Read the model definition and answer for the solid it produces. Units are mm, in the model's axes. A direction names the side the tool comes from. Coordinates: 2 decimals unless noted, no trailing zeros. Write each loop counter-clockwise with the first axis right and the second up, starting at its lowest first coordinate (ties: lowest second). Pieces come first, ordered by that corner, then holes. Notation, with made-up numbers: (12.5, 83.5) -> (42.5, 83.5) arc R5 cw to (42.5, 90.5) -> close; hole circle Ø3 at (-12.75, 77). An arc over 180 degrees is marked (long way). Answer as a JSON object with one key per item and string values. Group by question number.
(1) For a pull along Y with two mould halves and no side action, classify faces 4 (the face through (150.266, 29.026, 67.55)), 5 (the face through (150, 660.4, 89)), 6 (the face through (304.8, 326, 84)) as +Y half, -Y half, draft (parallel to the pull), parting line (faces both ways), or undercut.
(2) Which of the six approach directions +Z, -Z, +X, -X, +Y, -Y give full straight-line access (tool end or side, diameter ignored) to faces 1 (the face through (150.266, 273.576, 66.708)), 2 (the face through (150, 13, 56.872)), 3 (the face through (150, 585, 69.85))?
(3) Straight lines are drawn through the part: L1, parallel to Y at x = 57.5, z = 60; L2, parallel to Z at x = 71, y = 619; L3, parallel to Y at x = 237, z = 50. For each, find the intervals that lie inside material, in ascending order.
(4) Flat-ended cylindrical pins translate along their axes: P1, Ø1.5, axis at x = 97, z = 37.5, coming from the -Y side; P2, Ø1.5, axis at x = 111.5, z = 45.5, coming from the -Y side; P3, Ø20.5, axis at x = 89.5, y = 18, coming from the -Z side. Find the tip coordinate at first contact, or state that the pin passes through.
(5) Find section B-B (y = 566). Give the vertices of the cut face in (x, z).
(6) Find section A-A (x = 264.5). Give the vertices of the cut face in (y, z), then the cut area to 3 significant figures.
(7) Find section C-C (z = 44.5). Give the vertices of the cut face in (x, y), then the cut area to 3 significant figures.
from build123d import *

# Parameters (mm, degrees)
F1_W     = 660.4
F1_H     = 107.95
F2_DEPTH = 304.8
F3_DEPTH = 304.801


with BuildPart() as f2:
    # F1 (on Right) → F2 (new body)
    with BuildSketch(Plane.YZ):
        with Locations((330.2, 53.975)):
            Rectangle(F1_W, F1_H)
    extrude(amount=F2_DEPTH)

    # F0 (on Right) → F3 (cut, through all)
    with BuildSketch(Plane.YZ):
        with BuildLine():
            Line((0, 0), (25.4, 0))
            Line((25.4, 0), (635, 0))
            Line((635, 0), (660.4, 0))
            Line((660.4, 0), (660.4, 69.85))
            Line((660.4, 69.85), (635, 69.85))
            Line((635, 69.85), (508, 69.85))
            ThreePointArc((508, 69.85), (501.120084, 68.473081), (495.3, 64.554436))
            ThreePointArc((495.3, 64.554436), (387.828804, 19.05896), (279.4, 62.222496))
            ThreePointArc((279.4, 62.222496), (273.485985, 66.762175), (266.7, 69.85))
            ThreePointArc((266.7, 69.85), (152.689214, 88.843713), (38.1, 73.726423))
            ThreePointArc((38.1, 73.726423), (28.93043, 67.423949), (25.4, 56.872255))
            Line((25.4, 56.872255), (0, 56.872255))
            Line((0, 56.872255), (0, 0))
        make_face()
    extrude(amount=F3_DEPTH, mode=Mode.SUBTRACT)


solid = f2.part
Results below:
{
 "1": {"face 4": "undercut", "face 5": "+Y half", "face 6": "draft"},
 "2": {"face 1": "-Z, +X, -X", "face 2": "-Z, +X, -X, -Y", "face 3": "-Z, +X, -X, +Y"},
 "3": {"L1": "y = 0 to 25.68, 281.75 to 490.59", "L2": "z = 69.85 to 107.95", "L3": "y = 293.7 to 478.64"},
 "4": {"P1": "stops at y = 311.81", "P2": "stops at y = 298.9", "P3": "stops at z = 56.87"},
 "5": {"outline": "(0, 69.85) -> (304.8, 69.85) -> (304.8, 107.95) -> (0, 107.95) -> close"},
 "6": {"outline": "(0, 56.87) -> (25.4, 56.87) arc R17.53 cw to (38.1, 73.73) arc R391.58 cw to (266.7, 69.85) arc R32.82 cw to (279.4, 62.22) arc R153.61 ccw to (495.3, 64.55) arc R17.88 cw to (508, 69.85) -> (660.4, 69.85) -> (660.4, 107.95) -> (0, 107.95) -> close", "area": "30,500 mm2"},
 "7": {"outline": "(0, 301.49) -> (304.8, 301.49) -> (304.8, 470.85) -> (0, 470.85) -> close", "area": "51,600 mm2"}
}
